Read the model definition and answer for the solid it produces. Units are mm, in the model's axes. A direction names the side the tool comes from. Round coordinates to 2 decimals unless told otherwise and drop trailing zeros. Order: outer loops, then holes, each group sorted by start corner. A loop starts at its lowest first (then second) coordinate and runs counter-clockwise, first axis right, second up. Notation, with made-up numbers: (83.5, 3) - (88.5, 3) arc R27 ccw to (88.5, 20) - close; hole circle Ø8 at (61, 52). An arc over 180 degrees is marked (long way). Answer as a JSON object with one key per item and string values. Group by question number.
Q1. A cutting plane is placed at B-B on z = 5.5. Count the separate pieces of the cut face and the enclosed holes in it, and give its area (3 significant figures).
Q2. A tool of negligible diameter and unlimited length cuts with its end or side. For faces 4 (the cylindrical face through (-14.896, 14.762, 6.198)), 5 (the cylindrical face through (3.05, -1.26, 1.23)), from which of +Z, -Z, +X, -X, +Y, -Y can it reach the whole face along a straight path? Write none if from no direction.
Q3. Given pin 1 Ø2 at (y, z) = (-14, 8) entering from -X; pin 2 Ø1.5 at (y, z) = (-4, 3.5) entering from -X; pin 3 Ø5 at (x, z) = (10, 8) entering from -Y, each flat-ended and moving along its own axis, determine where each tip first touches the part or whether it passes through.
Q4. The mould has two halves that part along Y. Classify faces 1 (the flat face through (0, -5, 0)), 2 (the cylindrical face through (16.561, -13.315, 6.198)), 3 (the cylindrical face through (2.55, -18.53, 6.2)): pulls with the +Y half, pulls with the -Y half, needs draft (parallel to the pull), parting line crosses it, or undercut.
Q5. A cutting plane is placed at A-A on x = 0. Determine the outline of the cut face in (y, z), and give its area (3 significant figures).
Q6. A cutting plane is placed at D-D on y = -16. Determine the outline of the cut face in (x, z), and give its area (3 significant figures).
Q7. A cutting plane is placed at C-C on y = 1. Determine the outline of the cut face in (x, z).
Q8. Consider line 1 (Y direction, x = 0, z = 1.1); line 2 (Z direction, x = -12.5, y = 6); line 3 (Y direction, x = -19, z = 5.25). Determine where each line is inside the solid, lowest interval first.
```python
from build123d import *

# Parameters (mm, degrees)
F0_R     = 22.5
F0_R_2   = 3.302
F1_DEPTH = 2.5
F2_R     = 1.5
F3_DEPTH = 7.5


with BuildPart() as f1:
    # F0 (on Top) → F1 (new body)
    with BuildSketch(Plane.XY):
        Circle(F0_R)
        Circle(F0_R_2, mode=Mode.SUBTRACT)
    extrude(amount=F1_DEPTH)

    # F2 (on face) → F3 (join)
    with BuildSketch(Plane.XY.offset(2.5)):
        with Locations((0, 19.88579)):
            Circle(F2_R)
        with Locations((-7.183576, 18.542947)):
            Circle(F2_R)
        with Locations((-13.39697, 14.695776)):
            Circle(F2_R)
        with Locations((-17.801029, 8.863859)):
            Circle(F2_R)
        with Locations((-19.800961, 1.834829)):
            Circle(F2_R)
        with Locations((-19.126663, -5.442005)):
            Circle(F2_R)
        with Locations((-15.869203, -11.983866)):
            Circle(F2_R)
        with Locations((-10.46852, -16.90724)):
            Circle(F2_R)
        with Locations((-3.654004, -19.547197)):
            Circle(F2_R)
        with Locations((3.654004, -19.547197)):
            Circle(F2_R)
        with Locations((10.46852, -16.90724)):
            Circle(F2_R)
        with Locations((15.869203, -11.983866)):
            Circle(F2_R)
        with Locations((19.126663, -5.442005)):
            Circle(F2_R)
        with Locations((19.800961, 1.834829)):
            Circle(F2_R)
        with Locations((17.801029, 8.863859)):
            Circle(F2_R)
        with Locations((13.39697, 14.695776)):
            Circle(F2_R)
        with Locations((7.183576, 18.542947)):
            Circle(F2_R)
    extrude(amount=F3_DEPTH)


solid = f1.part
```
Result set:
{
 "1": {"separate pieces": "17", "enclosed holes": "0", "area": "120 mm²"},
 "2": {"face 4": "+Z", "face 5": "+Z, -Z"},
 "3": {"pin 1": "stops at x = -16.97", "pin 2": "stops at x = -20.46", "pin 3": "stops at y = -18.41"},
 "4": {"face 1": "needs draft", "face 2": "undercut", "face 3": "parting line crosses it"},
 "5": {"outline": "(-22.5, 0) - (-3.3, 0) - (-3.3, 2.5) - (-22.5, 2.5) - close; (3.3, 0) - (22.5, 0) - (22.5, 2.5) - (21.39, 2.5) - (21.39, 10) - (18.39, 10) - (18.39, 2.5) - (3.3, 2.5) - close", "area": "118 mm²"},
 "6": {"outline": "(-15.82, 0) - (15.82, 0) - (15.82, 2.5) - (11.66, 2.5) - (11.66, 10) - (9.27, 10) - (9.27, 2.5) - (-9.27, 2.5) - (-9.27, 10) - (-11.66, 10) - (-11.66, 2.5) - (-15.82, 2.5) - close", "area": "115 mm²"},
 "7": {"outline": "(-22.48, 0) - (-3.15, 0) - (-3.15, 2.5) - (-18.55, 2.5) - (-18.55, 10) - (-21.05, 10) - (-21.05, 2.5) - (-22.48, 2.5) - close; (3.15, 0) - (22.48, 0) - (22.48, 2.5) - (21.05, 2.5) - (21.05, 10) - (18.55, 10) - (18.55, 2.5) - (3.15, 2.5) - close"},
 "8": {"line 1": "y = -22.5 to -3.3, 3.3 to 22.5", "line 2": "z = 0 to 2.5", "line 3": "y = -6.94 to -3.95, 0.57 to 3.1, 7.96 to 9.77"}
}
